```python
from build123d import *

# Parameters (mm, degrees)
F0_W          = 34
F0_H          = 94
F0_R          = 1.5
F0_R_2        = 2.15
F1_DEPTH      = 8
F2_W          = 8
F2_H          = 8
F3_DEPTH      = 3
F4_W          = 8
F4_H          = 5.470946
F5_DEPTH      = 100
F5_DEPTH_BACK = 28


with BuildPart() as f1:
    # F0 (on Top) → F1 (new body)
    with BuildSketch(Plane.XY):
        Rectangle(F0_W, F0_H)
        with Locations((-13, -43)):
            Circle(F0_R, mode=Mode.SUBTRACT)
        with Locations((13, -43)):
            Circle(F0_R, mode=Mode.SUBTRACT)
        with Locations((0, -23)):
            Circle(F0_R_2, mode=Mode.SUBTRACT)
        with Locations((-13, 43)):
            Circle(F0_R, mode=Mode.SUBTRACT)
        Circle(F0_R_2, mode=Mode.SUBTRACT)
        with Locations((0, 23)):
            Circle(F0_R_2, mode=Mode.SUBTRACT)
        with Locations((13, 43)):
            Circle(F0_R, mode=Mode.SUBTRACT)
    extrude(amount=F1_DEPTH)

    # F2 (on Top) → F3 (cut)
    with BuildSketch(Plane.XY):
        with Locations((-13, 43)):
            Rectangle(F2_W, F2_H)
        with Locations((13, 43)):
            Rectangle(F2_W, F2_H)
        with Locations((-13, -43)):
            Rectangle(F2_W, F2_H)
        with Locations((13, -43)):
            Rectangle(F2_W, F2_H)
    extrude(amount=F3_DEPTH, mode=Mode.SUBTRACT)

    # F4 (on Front) → F5 (cut, two sides)
    with BuildSketch(Plane.XZ) as f5_sk:
        with Locations((0, 1.264527)):
            Rectangle(F4_W, F4_H)
    extrude(amount=F5_DEPTH, mode=Mode.SUBTRACT)
    extrude(f5_sk.sketch, amount=-F5_DEPTH_BACK, mode=Mode.SUBTRACT)


solid = f1.part
```
Check sheet for the modelled part. Datum: model origin and axes. Units: mm. A direction names the side the tool comes from. Round coordinates to 2 decimals unless told otherwise and drop trailing zeros. Loops run counter-clockwise (first coordinate to the right, second up) from the corner with the lowest first, then second, coordinate; pieces in that order, holes last. Notation, with made-up numbers: M 73,52.25 L 92,52.25 A24 ccw 92,66.25 Z; hole C -26,-29 d6. An arc over 180 degrees is marked long. Answer as a JSON object with one key per item and string values.
1. Access from +Z, -Z, +X, -X, +Y, -Y to the whole of each face (thin tool, end or side, straight path). Record for faces 1 (the flat face through (-13, -39, 1)), 2 (the flat face through (0, -9, 4)), 3 (the flat face through (13, 41, 3)), 4 (the flat face through (-13, 41, 3)).
Reply:
{"face 1": "-Z, -X, -Y", "face 2": "-Z, -Y", "face 3": "-Z, +X, +Y", "face 4": "-Z, -X, +Y"}
2. Section check C-C (y = 23). Record the boundary of the cut face in (x, z), plus the area to 3 significant figures.
Reply:
{"outline": "M -17,0 L -4,0 L -4,4 L -2.15,4 L -2.15,8 L -17,8 Z; M 2.15,4 L 4,4 L 4,0 L 17,0 L 17,8 L 2.15,8 Z", "area": "223 mm²"}
3. Section check D-D (x = 13). Record the boundary of the cut face in (y, z), plus the area to 3 significant figures.
Reply:
{"outline": "M -47,3 L -44.5,3 L -44.5,8 L -47,8 Z; M -41.5,3 L -39,3 L -39,0 L 39,0 L 39,3 L 41.5,3 L 41.5,8 L -41.5,8 Z; M 44.5,3 L 47,3 L 47,8 L 44.5,8 Z", "area": "674 mm²"}
4. Gauge pin test, flat ends, axial feed: P1, Ø2.5, axis at x = -13.5, y = -43, coming from the -Z side; P2, Ø1.5, axis at y = 41, z = 1.5, coming from the -X side; P3, Ø0.9, axis at x = 11, z = 1.5, coming from the +Y side. Record the tip position at first contact, or that the pin passes through.
Reply:
{"P1": "stops at z = 3", "P2": "stops at x = -9", "P3": "stops at y = 39"}
5. Section check A-A (y = -43). Record the boundary of the cut face in (x, z), plus the area to 3 significant figures.
Reply:
{"outline": "M -17,3 L -14.5,3 L -14.5,8 L -17,8 Z; M -11.5,3 L -9,3 L -9,0 L -4,0 L -4,4 L 4,4 L 4,0 L 9,0 L 9,3 L 11.5,3 L 11.5,8 L -11.5,8 Z; M 14.5,3 L 17,3 L 17,8 L 14.5,8 Z", "area": "162 mm²"}
6. Scan lines: line 1 (Y direction, x = 13, z = 4.95); line 2 (X direction, y = -30, z = 1); line 3 (X direction, y = 23, z = 5.8). Record each from-to range of solid material in increasing order.
Reply:
{"line 1": "y = -47 to -44.5, -41.5 to 41.5, 44.5 to 47", "line 2": "x = -17 to -4, 4 to 17", "line 3": "x = -17 to -2.15, 2.15 to 17"}
7. Section check B-B (x = 0). Record the boundary of the cut face in (y, z), plus the area to 3 significant figures.
Reply:
{"outline": "M -47,4 L -25.15,4 L -25.15,8 L -47,8 Z; M -20.85,4 L -2.15,4 L -2.15,8 L -20.85,8 Z; M 2.15,4 L 20.85,4 L 20.85,8 L 2.15,8 Z; M 25.15,4 L 28,4 L 28,0 L 47,0 L 47,8 L 25.15,8 Z", "area": "400 mm²"}
8. Mould release check, pull along Y, two halves, no side actions. Record for faces 5 (the cylindrical face through (-0.47, 20.9, 5.97)), 6 (the flat face through (0, 47, 5)), 7 (the flat face through (-8, 1, 0)): pulls with the +Y half, pulls with the -Y half, needs draft (parallel to the pull), parting line crosses it, or undercut.
Reply:
{"face 5": "undercut", "face 6": "pulls with the +Y half", "face 7": "needs draft"}
